Design review of the part built by this model. Coordinates are the model's own, in mm. A direction names the side the tool comes from. Coordinates: 2 decimals unless noted, no trailing zeros. Loops run counter-clockwise (first coordinate to the right, second up) from the corner with the lowest first, then second, coordinate; pieces in that order, holes last. Notation, with made-up numbers: (71, 53.5) -> (128, 53.5) arc R7 ccw to (128, 65.5) -> close; hole circle Ø11 at (-22, -6.75). An arc over 180 degrees is marked (long way). One line per item, written item: value. Start each with the question number.
1. Add section C-C on y = 10. Write out the cut boundary in (x, z).
2. Add section B-B on z = 30. Write out the cut boundary in (x, y), plus the area to 3 significant figures.
3. Insertion check: pin 1 (5 mm diameter, centred on x = 9, z = 37, fed in from -Y); pin 2 (2 mm diameter, centred on x = 17, z = 24, fed in from +Y); pin 3 (12 mm diameter, centred on x = 19, y = 32, fed in from -Z); pin 4 (1.5 mm diameter, centred on x = 2.5, y = 4, fed in from +Z). Each pin has a flat end and moves straight along its axis. Give the tip position at first contact, or say it passes through.
4. Machinability: for faces 1 (the flat face through (13.315, 32.689, 37.535)), 2 (the flat face through (0, 10, 20)), 3 (the cylindrical face through (21, 33, 28)), which of the approach directions +Z, -Z, +X, -X, +Y, -Y give a long, thin tool a straight path to every point of the face, cutting with its end or side? Answer none if there is none.
5. Add section D-D on x = 10. Write out the cut boundary in (y, z), plus the area to 3 significant figures.
6. Add section A-A on y = 15.5. Write out the cut boundary in (x, z).
7. For probe 1 along X at (y, z) = (18.5, 21.5); probe 2 along Y at (x, z) = (21.3, 30); probe 3 along X at (y, z) = (24, 24), list the stretches that pass through material, from the lowest coordinate up.
8. Draft analysis for pull direction Y (two halves, no side actions). For faces 4 (the flat face through (10, 31, 34)), 5 (the flat face through (13, 27, 40)), 6 (the flat face through (10, 25, 23)), state which applies: pulls with the +Y half, pulls with the -Y half, needs draft (parallel to the pull), parting line crosses it, or undercut.
```python
from build123d import *

# Parameters (mm, degrees)
EXTRUDE_1_DEPTH     = 40
CUT_EXTRUDE_1_DEPTH = 61.373835392
SKETCH_3_R          = 2.55
CUT_EXTRUDE_2_DEPTH = 61.373835392
CUT_EXTRUDE_3_DEPTH = 5
SKETCH_6_R          = 2.55
CUT_EXTRUDE_4_DEPTH = 1


with BuildPart() as part:
    # Эскиз1 → Бобышка-Вытянуть1 (new body)
    with BuildSketch(Plane.XY):
        with BuildLine():
            Line((0, 0), (0, 20))
            ThreePointArc((0, 20), (1.464466094, 23.535533906), (5, 25))
            Line((5, 25), (15, 25))
            ThreePointArc((15, 25), (18.535533906, 23.535533906), (20, 20))
            Line((20, 20), (20, 0))
            Line((20, 0), (23, 0))
            Line((23, 0), (23, 27))
            ThreePointArc((23, 27), (20.071067812, 34.071067812), (13, 37))
            Line((13, 37), (7, 37))
            ThreePointArc((7, 37), (-0.071067812, 34.071067812), (-3, 27))
            Line((-3, 27), (-3, 0))
            Line((-3, 0), (0, 0))
        make_face()
    extrude(amount=EXTRUDE_1_DEPTH)

    # Эскиз2 → Вырез-Вытянуть1 (cut, through all)
    with BuildSketch(Plane(origin=(23, 0, 0), x_dir=(0, 0, -1), z_dir=(1, 0, 0))):
        Polygon((0, 20), (-25, 37), (0, 37), align=None)
    extrude(amount=-CUT_EXTRUDE_1_DEPTH, mode=Mode.SUBTRACT)

    # Эскиз3 → Вырез-Вытянуть2 (cut, through all)
    with BuildSketch(Plane(origin=(23, 0, 0), x_dir=(0, 0, -1), z_dir=(1, 0, 0))):
        with Locations((-30, 10)):
            Circle(SKETCH_3_R)
        with Locations((-10, 10)):
            Circle(SKETCH_3_R)
    extrude(amount=-CUT_EXTRUDE_2_DEPTH, mode=Mode.SUBTRACT)

    # Эскиз4 → Вырез-Вытянуть3 (cut)
    with BuildSketch(Plane.XY.offset(40)):
        Polygon((5.6, 30.810511777), (7.8, 27), (12.2, 27), (14.4, 30.810511777), (12.2, 34.621023553), (7.8, 34.621023553), align=None)
    extrude(amount=-CUT_EXTRUDE_3_DEPTH, mode=Mode.SUBTRACT)

    # Эскиз6 → Вырез-Вытянуть4 (cut)
    with BuildSketch(Plane.XY.offset(35)):
        with Locations((10, 30.810511777)):
            Circle(SKETCH_6_R)
    extrude(amount=-CUT_EXTRUDE_4_DEPTH, mode=Mode.SUBTRACT)


solid = part.part
```
Worked answers:
1. outline: (-3, 0) -> (0, 0) -> (0, 7.45) -> (-3, 7.45) -> close; (-3, 12.55) -> (0, 12.55) -> (0, 27.45) -> (-3, 27.45) -> close; (-3, 32.55) -> (0, 32.55) -> (0, 40) -> (-3, 40) -> close; (20, 0) -> (23, 0) -> (23, 7.45) -> (20, 7.45) -> close; (20, 12.55) -> (23, 12.55) -> (23, 27.45) -> (20, 27.45) -> close; (20, 32.55) -> (23, 32.55) -> (23, 40) -> (20, 40) -> close
2. outline: (-3, 0) -> (0, 0) -> (0, 7.45) -> (-3, 7.45) -> close; (-3, 12.55) -> (0, 12.55) -> (0, 20) arc R5 cw to (5, 25) -> (15, 25) arc R5 cw to (20, 20) -> (20, 12.55) -> (23, 12.55) -> (23, 27) arc R10 ccw to (13, 37) -> (7, 37) arc R10 ccw to (-3, 27) -> close; (20, 0) -> (23, 0) -> (23, 7.45) -> (20, 7.45) -> close
2. area: 399 mm²
3. pin 1: stops at y = 25
3. pin 2: stops at y = 36.52
3. pin 3: stops at z = 8.82
3. pin 4: passes through
4. face 1: +Z
4. face 2: +Z, -Z, -Y
4. face 3: +Z, -Z, +X, +Y
5. outline: (25, 7.35) -> (37, 25) -> (37, 40) -> (34.62, 40) -> (34.62, 35) -> (33.36, 35) -> (33.36, 34) -> (28.26, 34) -> (28.26, 35) -> (27, 35) -> (27, 40) -> (25, 40) -> close
5. area: 243 mm²
6. outline: (-3, 0) -> (0, 0) -> (0, 40) -> (-3, 40) -> close; (20, 0) -> (23, 0) -> (23, 40) -> (20, 40) -> close
7. probe 1: x = -3 to 0, 20 to 23
7. probe 2: y = 0 to 7.45, 12.55 to 32.58
7. probe 3: x = -3 to 2, 18 to 23
8. face 4: undercut
8. face 5: needs draft
8. face 6: pulls with the -Y half
